Verification items for the finished model (mm, model axes). A direction names the side the tool comes from. Round coordinates to 2 decimals unless told otherwise and drop trailing zeros. Order: outer loops, then holes, each group sorted by start corner. A loop starts at its lowest first (then second) coordinate and runs counter-clockwise, first axis right, second up. Notation, with made-up numbers: M 43,20.25 L 48,20.25 A16 cw 48,37.25 Z; hole C 58,-25 d10. An arc over 180 degrees is marked long. Return JSON: item names as keys, results as strings. Group by question number.
from build123d import *

# Parameters (mm, degrees)
SKETCH1_W               = 310
SKETCH1_H               = 310
BOSS_EXTRUDE1_DEPTH     = 6
BOSS_EXTRUDE2_DEPTH     = 6
SKETCH4_R               = 51.5
CUT_EXTRUDE1_DEPTH      = 439.570404838
SKETCH10_R              = 10
CORNER_CORD_HOLE_DEPTH  = 439.570404838
SKETCH11_R              = 2
CUT_EXTRUDE5_DEPTH      = 439.570404838
SKETCH12_W              = 25
SKETCH12_H              = 10
BOSS_EXTRUDE3_DEPTH     = 6.5
SKETCH13_W              = 25
SKETCH13_H              = 112
BOSS_EXTRUDE4_DEPTH     = 8
CUT_EXTRUDE6_DEPTH      = 440.206386566
CUT_EXTRUDE6_DEPTH_BACK = 440.206386566
SKETCH14_R              = 1.5


with BuildPart() as part:
    # Sketch1 → Boss-Extrude1 (new body)
    with BuildSketch(Plane.XY):
        with Locations((155, -155)):
            Rectangle(SKETCH1_W, SKETCH1_H)
    extrude(amount=BOSS_EXTRUDE1_DEPTH)

    # Sketch3 → Boss-Extrude2 (add)
    with BuildSketch(Plane.XY.offset(6)):
        Polygon((302, -8), (302, -33), (302, -277), (302, -302), (277, -302), (33, -302), (8, -302), (8, -277), (8, -33), (8, -8), (33, -8), (277, -8), align=None)
        Polygon((268.286796564, -20.5), (223.286796564, -65.5), (86.713203436, -65.5), (41.713203436, -20.5), align=None, mode=Mode.SUBTRACT)
        Polygon((20.5, -41.713203436), (65.5, -86.713203436), (65.5, -223.286796564), (20.5, -268.286796564), align=None, mode=Mode.SUBTRACT)
        Polygon((41.713203436, -289.5), (86.713203436, -244.5), (223.286796564, -244.5), (268.286796564, -289.5), align=None, mode=Mode.SUBTRACT)
        Polygon((289.5, -41.713203436), (244.5, -86.713203436), (244.5, -223.286796564), (289.5, -268.286796564), align=None, mode=Mode.SUBTRACT)
    extrude(amount=BOSS_EXTRUDE2_DEPTH)

    # Sketch4 → Cut-Extrude1 (cut, through all)
    with BuildSketch(Plane.XY.offset(12)):
        with Locations((155, -155)):
            Circle(SKETCH4_R)
    extrude(amount=-CUT_EXTRUDE1_DEPTH, mode=Mode.SUBTRACT)

    # Sketch10 → corner cord hole (cut, through all)
    with BuildSketch(Plane(origin=(0, 0, 0), x_dir=(-1, 0, 0), z_dir=(0, 0, -1))):
        with Locations((-252.5, -52.5)):
            Circle(SKETCH10_R)
    extrude(amount=-CORNER_CORD_HOLE_DEPTH, mode=Mode.SUBTRACT)

    # Sketch11 → Cut-Extrude5 (cut, through all)
    with BuildSketch(Plane(origin=(0, 0, 0), x_dir=(-1, 0, 0), z_dir=(0, 0, -1))):
        with Locations((-55, -55)):
            Circle(SKETCH11_R)
        with Locations((-55, -255)):
            Circle(SKETCH11_R)
    extrude(amount=-CUT_EXTRUDE5_DEPTH, mode=Mode.SUBTRACT)

    # Sketch12 → Boss-Extrude3 (add)
    with BuildSketch(Plane(origin=(0, 0, 0), x_dir=(-1, 0, 0), z_dir=(0, 0, -1))):
        with Locations((-272.5, -104)):
            Rectangle(SKETCH12_W, SKETCH12_H)
        with Locations((-272.5, -206)):
            Rectangle(SKETCH12_W, SKETCH12_H)
    extrude(amount=BOSS_EXTRUDE3_DEPTH)

    # Sketch13 → Boss-Extrude4 (add)
    with BuildSketch(Plane(origin=(0, 0, -6.5), x_dir=(-1, 0, 0), z_dir=(0, 0, -1))):
        with Locations((-272.5, -155)):
            Rectangle(SKETCH13_W, SKETCH13_H)
    extrude(amount=BOSS_EXTRUDE4_DEPTH)

    # Sketch14 → Cut-Extrude6 (cut, two sides: drawn at the far end of the back side and taken through both)
    with BuildSketch(Plane.XY.offset(12).offset(-CUT_EXTRUDE6_DEPTH_BACK)):
        with Locations((33, -33)):
            Circle(SKETCH14_R)
        with Locations((277, -33)):
            Circle(SKETCH14_R)
        with Locations((277, -277)):
            Circle(SKETCH14_R)
        with Locations((33, -277)):
            Circle(SKETCH14_R)
    extrude(amount=CUT_EXTRUDE6_DEPTH + CUT_EXTRUDE6_DEPTH_BACK, mode=Mode.SUBTRACT)


solid = part.part
1. Cross-section at C-C (x = 232). Enter the section's corners in (y, z), plus the area to 3 significant figures.
2. Thickness scan on line 1 along Y through (x, z) = (33, 3); line 2 along X through (y, z) = (-145, 8.75); line 3 along X through (y, z) = (-255, 5). Record the ranges inside material, lowest first. Write a range as from..to.
3. Cross-section at A-A (x = 155). Enter the section's corners in (y, z).
4. Access from +Z, -Z, +X, -X, +Y, -Y to the whole of each face (thin tool, end or side, straight path). Record for faces 1 (the face through (260, -156, -9)), 2 (the face through (64.528, -43.315, 8.958)), 3 (the face through (273, -99, -7)), 4 (the face through (273, -154, -6.5)).
5. Go/stop test with flat-tipped pins: pin 1 (4 mm diameter, centred on y = -205, z = -11.5, fed in from +X); pin 2 (7 mm diameter, centred on y = -146, z = -10, fed in from -X); pin 3 (13.5 mm diameter, centred on x = 191.5, y = -36.5, fed in from +Z). Record where each tip stops, or that it passes through.
6. Draft check along Y on faces 5 (the face through (43, -153, 6)), 6 (the face through (273, -211, -7)), 7 (the face through (273, -154, -14.5)). Enter one of: +Y half, -Y half, draft (parallel to the pull), parting line (faces both ways), or undercut.
7. Cross-section at B-B (y = -144.5). Enter the section's corners in (x, z), plus the area to 3 significant figures.
Computed:
{
 "1": {"outline": "M -310,0 L 0,0 L 0,6 L -8,6 L -8,12 L -20.5,12 L -20.5,6 L -56.79,6 L -56.79,12 L -253.21,12 L -253.21,6 L -289.5,6 L -289.5,12 L -302,12 L -302,6 L -310,6 Z", "area": "3,190 mm²"},
 "2": {"line 1": "y = -310..-278.5, -275.5..-34.5, -31.5..0", "line 2": "x = 8..20.5, 65.5..104.48, 205.52..244.5, 289.5..302", "line 3": "x = 0..53, 57..310"},
 "3": {"outline": "M -310,0 L -206.5,0 L -206.5,12 L -244.5,12 L -244.5,6 L -289.5,6 L -289.5,12 L -302,12 L -302,6 L -310,6 Z; M -103.5,0 L 0,0 L 0,6 L -8,6 L -8,12 L -20.5,12 L -20.5,6 L -65.5,6 L -65.5,12 L -103.5,12 Z"},
 "4": {"face 1": "-Z, -X, +Y, -Y", "face 2": "+Z", "face 3": "-Z, +X, -X, +Y", "face 4": "+X, -X"},
 "5": {"pin 1": "stops at x = 285", "pin 2": "stops at x = 260", "pin 3": "stops at z = 6"},
 "6": {"face 5": "undercut", "face 6": "-Y half", "face 7": "draft"},
 "7": {"outline": "M 0,0 L 104.58,0 L 104.58,12 L 65.5,12 L 65.5,6 L 20.5,6 L 20.5,12 L 8,12 L 8,6 L 0,6 Z; M 205.42,0 L 310,0 L 310,6 L 302,6 L 302,12 L 289.5,12 L 289.5,6 L 244.5,6 L 244.5,12 L 205.42,12 Z; M 260,-14.5 L 285,-14.5 L 285,-6.5 L 260,-6.5 Z", "area": "2,070 mm²"}
}
